from build123d import *

# Parameters (mm, degrees)
EXTRUDE_1_DEPTH     = 40
SKETCH_2_R          = 1.75
CUT_EXTRUDE_1_DEPTH = 69.135893624
CUT_EXTRUDE_2_DEPTH = 69.135893624
FILLET_1_R          = 20
FILLET_2_R          = 20
SKETCH_7_R          = 1.5
CUT_EXTRUDE_3_DEPTH = 69.135893624


with BuildPart() as part:
    # 草图1 → 凸台-拉伸1 (new body)
    with BuildSketch(Plane.XY):
        with BuildLine():
            Line((0, 38.5), (0, 2))
            ThreePointArc((0, 2), (0.585786438, 0.585786438), (2, 0))
            Line((2, 0), (39.5, 0))
            Line((39.5, 0), (39.5, -2))
            Line((39.5, -2), (0, -2))
            ThreePointArc((0, -2), (-1.414213562, -1.414213562), (-2, 0))
            Line((-2, 0), (-2, 38.5))
            Line((-2, 38.5), (0, 38.5))
        make_face()
    extrude(amount=EXTRUDE_1_DEPTH)

    # 草图2 → 切除-拉伸1 (cut, through all)
    with BuildSketch(Plane(origin=(0, 0, 0), x_dir=(1, 0, 0), z_dir=(0, 1, 0))):
        with Locations(Location((5.75, -32, 0), (0, 0, 270))):
            Circle(SKETCH_2_R)
        with Locations(Location((35.75, -32, 0), (0, 0, 90))):
            Circle(SKETCH_2_R)
        with Locations(Location((5.75, -8, 0), (0, 0, 90))):
            Circle(SKETCH_2_R)
        with Locations(Location((35.75, -8, 0), (0, 0, 270))):
            Circle(SKETCH_2_R)
    extrude(amount=-CUT_EXTRUDE_1_DEPTH, mode=Mode.SUBTRACT)

    # 草图3 → 切除-拉伸2 (cut, through all)
    with BuildSketch(Plane(origin=(0, 0, 0), x_dir=(0, 0, -1), z_dir=(1, 0, 0))):
        with BuildLine():
            Line((-14, 28.5), (-14, 20.25))
            ThreePointArc((-14, 20.25), (-20, 14.25), (-26, 20.25))
            Line((-26, 20.25), (-26, 28.5))
            ThreePointArc((-26, 28.5), (-20, 34.5), (-14, 28.5))
        make_face()
    extrude(amount=-CUT_EXTRUDE_2_DEPTH, mode=Mode.SUBTRACT)

    # 圆角1
    fillet_1_edges = [part.edges().sort_by_distance(p)[0] for p in [
        (-1, 38.5, 40),
    ]]
    fillet(fillet_1_edges, radius=FILLET_1_R)

    # 圆角2
    fillet_2_edges = [part.edges().sort_by_distance(p)[0] for p in [
        (-1, 38.5, 0),
    ]]
    fillet(fillet_2_edges, radius=FILLET_2_R - 0.0001)  # a hair under: the kernel refuses the full size

    # 草图7 → 切除-拉伸3 (cut, through all)
    with BuildSketch(Plane(origin=(0, 0, 0), x_dir=(0, 0, -1), z_dir=(1, 0, 0))):
        with Locations(Location((-28, 19.5, 0), (0, 0, 90))):
            Circle(SKETCH_7_R)
        with Locations(Location((-12, 19.5, 0), (0, 0, 270))):
            Circle(SKETCH_7_R)
    extrude(amount=-CUT_EXTRUDE_3_DEPTH, mode=Mode.SUBTRACT)


solid = part.part
Design review of the part built by this model. Coordinates are the model's own, in mm. A direction names the side the tool comes from. Round coordinates to 2 decimals unless told otherwise and drop trailing zeros. Write each loop counter-clockwise with the first axis right and the second up, starting at its lowest first coordinate (ties: lowest second). Pieces come first, ordered by that corner, then holes.
Item 1: Consider section A-A on z = 32. Give the boundary of the cut face in (x, y), and give its area (3 significant figures).
Item 2: Consider section C-C on z = 18. Give the boundary of the cut face in (x, y).
Item 3: For faces 1 (the flat face through (0, 16, 15)), 2 (the flat face through (14, -1, 40)), 3 (the flat face through (-1, 24, 14)), list the 3-axis set-ups (+Z, -Z, +X, -X, +Y, -Y) from which the entire face can be reached by the end or side of a thin tool; tool diameter is ignored.
Item 4: Consider section B-B on x = 35.75. Give the boundary of the cut face in (y, z), and give its area (3 significant figures).
Item 5: Consider section D-D on y = 19.5. Give the boundary of the cut face in (x, z).
Item 6: Draft analysis for pull direction Z (two halves, no side actions). For faces 4 (the flat face through (20, 0, 20)), 5 (the cylindrical face through (-1, 21, 12)), 6 (the cylindrical face through (-0.986, 32.797, 6.014)), state which applies: released by +Z, released by -Z, zero draft, split by the parting line, or undercut.
Item 7: Wall thickness on L1, parallel to X at y = -1, z = 32; L2, parallel to Y at x = 14.5, z = 25; L3, parallel to Z at x = -1.1, y = 19.5: over which ranges is each line inside the solid? List them lowest first.
Item 8: For pin 1 Ø12 at (y, z) = (21.5, 15.5) entering from -X; pin 2 Ø2 at (x, z) = (5.75, 32) entering from +Y; pin 3 Ø2 at (x, z) = (5, 27) entering from +Y; pin 4 Ø1.6 at (x, y) = (-1, 24) entering from -Z, all flat-tipped, find the tip position at first contact; note any pin that passes through.
Check values:
1. outline: (-2, 0) arc R2 ccw to (0, -2) - (4, -2) - (4, 0) - (2, 0) arc R2 cw to (0, 2) - (0, 34.5) - (-2, 34.5) - close; (7.5, -2) - (34, -2) - (34, 0) - (7.5, 0) - close; (37.5, -2) - (39.5, -2) - (39.5, 0) - (37.5, 0) - close
1. area: 138 mm2
2. outline: (-2, 0) arc R2 ccw to (0, -2) - (39.5, -2) - (39.5, 0) - (2, 0) arc R2 cw to (0, 2) - (0, 14.59) - (-2, 14.59) - close; (-2, 34.16) - (0, 34.16) - (0, 38.4) - (-2, 38.4) - close
3. face 1: +Z, -Z, +X, +Y
3. face 2: +Z, +X, -X, +Y, -Y
3. face 3: +X, -X
4. outline: (-2, 0) - (0, 0) - (0, 6.25) - (-2, 6.25) - close; (-2, 9.75) - (0, 9.75) - (0, 30.25) - (-2, 30.25) - close; (-2, 33.75) - (0, 33.75) - (0, 40) - (-2, 40) - close
4. area: 66.0 mm2
5. outline: (-2, 0.03) - (0, 0.03) - (0, 10.5) - (-2, 10.5) - close; (-2, 13.5) - (0, 13.5) - (0, 14.05) - (-2, 14.05) - close; (-2, 25.95) - (0, 25.95) - (0, 26.5) - (-2, 26.5) - close; (-2, 29.5) - (0, 29.5) - (0, 39.97) - (-2, 39.97) - close
6. face 4: zero draft
6. face 5: undercut
6. face 6: released by -Z
7. L1: x = -1.73 to 4, 7.5 to 34, 37.5 to 39.5
7. L2: y = -2 to 0
7. L3: z = 0.03 to 10.5, 13.5 to 14.05, 25.95 to 26.5, 29.5 to 39.97
8. pin 1: stops at x = -2
8. pin 2: passes through
8. pin 3: stops at y = 0
8. pin 4: stops at z = 0.56
